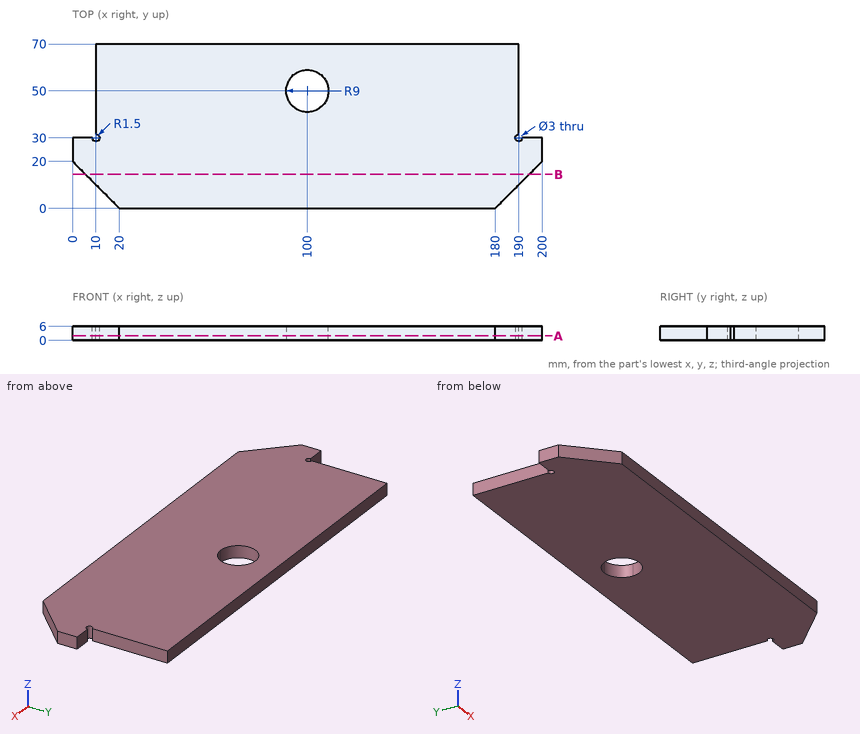
Geometry: see drawing. Coordinates: mm, zero at the bounding-box minimum. Give positions to 0.01 mm unless a question says otherwise; leave off trailing zeros. Loops run counter-clockwise (first coordinate to the right, second up) from the corner with the lowest first, then second, coordinate; pieces in that order, holes last. Notation, with made-up numbers: (19.25, 40) - (56.25, 40) arc R25 ccw to (56.25, 73) - close; hole circle Ø9 at (66.25, -6). An arc over 180 degrees is marked (long way). Answer as CSV lines item,"result". Start each with the question number.
1. Section B-B, the plane y = 14.5. Return loops of the section in (x, z).
2. Pin query (flat end, axial travel): P1, Ø3, axis at y = 48.5, z = 3.5, coming from the -X side; P2, Ø1.8, axis at x = 4, z = 3, coming from the +Y side; P3, Ø3, axis at y = 46, z = 2.5, coming from the +X side. Return the tip coordinate at first contact, or that it passes through.
3. Section A-A, the plane z = 2. Return loops of the section in (x, y), plus the area to 3 significant figures.
4. Ray query, L1, parallel to X at y = 49, z = 5; L2, parallel to X at y = 57, z = 4; L3, parallel to X at y = 35, z = 1. Return the intervals inside material, ascending.
Answers:
1,outline,"(5.5, 0) - (194.5, 0) - (194.5, 6) - (5.5, 6) - close"
2,P1,"stops at x = 10"
2,P2,"stops at y = 30"
2,P3,"stops at x = 190"
3,outline,"(0, 20) - (20, 0) - (180, 0) - (200, 20) - (200, 30) - (191.5, 30) arc R1.5 cw (long way) to (190, 31.5) - (190, 70) - (10, 70) - (10, 31.5) arc R1.5 cw (long way) to (8.5, 30) - (0, 30) - close; hole circle Ø18 at (100, 50)"
3,area,"12,500 mm2"
4,L1,"x = 10 to 91.06, 108.94 to 190"
4,L2,"x = 10 to 94.34, 105.66 to 190"
4,L3,"x = 10 to 190"
